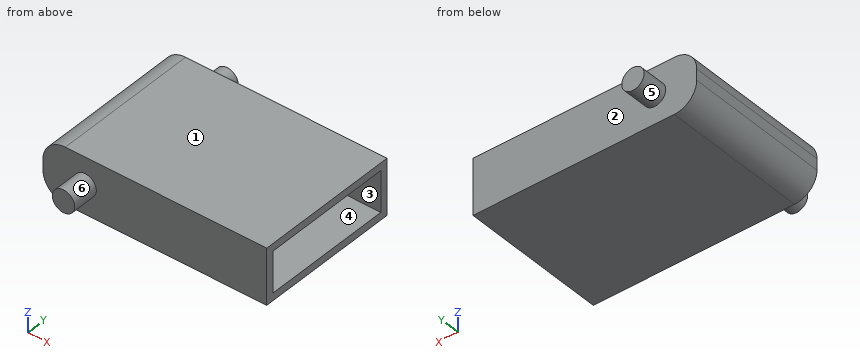
```python
from build123d import *

# Parameters (mm, degrees)
F1_DEPTH = 50
F2_T     = -2.54
F3_R     = 3.81
F4_DEPTH = 9
F5_R     = 3.81
F6_DEPTH = 9


with BuildPart() as f1:
    # F0 (on Front) → F1 (new body)
    with BuildSketch(Plane.XZ):
        with BuildLine():
            Line((31.366751, 9.340362), (-37.213249, 9.340362))
            ThreePointArc((-37.213249, 9.340362), (-42.601402, 7.108516), (-44.833249, 1.720362))
            Line((-44.833249, 1.720362), (-44.833249, -2.089638))
            ThreePointArc((-44.833249, -2.089638), (-42.601402, -7.477792), (-37.213249, -9.709638))
            Line((-37.213249, -9.709638), (31.366751, -9.709638))
            Line((31.366751, -9.709638), (31.366751, 9.340362))
        make_face()
    extrude(amount=F1_DEPTH)

    # F2
    f2_openings = [f1.faces().sort_by_distance(p)[0] for p in [
        (31.366751, -25, -0.184638),
    ]]
    offset(amount=F2_T, openings=f2_openings)

    # F3 (on face) → F4 (join)
    with BuildSketch(Plane.XZ.offset(50)):
        with Locations((-30.48, 0)):
            Circle(F3_R)
    extrude(amount=F4_DEPTH)

    # F5 (on face) → F6 (join)
    with BuildSketch(Plane(origin=(0, 0, 0), x_dir=(-1, 0, 0), z_dir=(0, 1, 0))):
        with Locations((30.48, 0)):
            Circle(F5_R)
    extrude(amount=F6_DEPTH)


solid = f1.part
```
Verification items for the finished model (mm, model axes). Face numbers are marked on the shaded views. A direction names the side the tool comes from. Coordinates: 2 decimals unless noted, no trailing zeros. Write each loop counter-clockwise with the first axis right and the second up, starting at its lowest first coordinate (ties: lowest second). Pieces come first, ordered by that corner, then holes. Notation, with made-up numbers: M 84,15 L 115,15 A19 cw 115,39 Z; hole C -9,-14.5 d10. An arc over 180 degrees is marked long. One line per item, written item: value.
Item 1: Access from +Z, -Z, +X, -X, +Y, -Y to the whole of each face (thin tool, end or side, straight path). Record for the marked faces 4, 5 and 6.
Check sheet entries:
face 4: +X
face 5: +Y
face 6: -Y
Item 2: Section check D-D, the plane x = -7. Record the boundary of the cut face in (y, z), plus the area to 3 significant figures.
Check sheet entries:
outline: M -50,-9.71 L 0,-9.71 L 0,9.34 L -50,9.34 Z; hole M -47.46,-7.17 L -2.54,-7.17 L -2.54,6.8 L -47.46,6.8 Z
area: 325 mm^2
Item 3: Section check C-C, the plane y = -19. Record the boundary of the cut face in (x, z).
Check sheet entries:
outline: M -44.83,-2.09 A7.62 ccw -37.21,-9.71 L 31.37,-9.71 L 31.37,-7.17 L -37.21,-7.17 A5.08 cw -42.29,-2.09 L -42.29,1.72 A5.08 cw -37.21,6.8 L 31.37,6.8 L 31.37,9.34 L -37.21,9.34 A7.62 ccw -44.83,1.72 Z
Item 4: Scan lines: line 1 along Y through (x, z) = (25, -0.5); line 2 along Z through (x, y) = (1, -10); line 3 along Y through (x, z) = (1, 7). Record each from-to range of solid material in increasing order.
Check sheet entries:
line 1: y = -50 to -47.46, -2.54 to 0
line 2: z = -9.71 to -7.17, 6.8 to 9.34
line 3: y = -50 to 0
Item 5: Section check B-B, the plane z = 0. Record the boundary of the cut face in (x, y), plus the area to 3 significant figures.
Check sheet entries:
outline: M -44.83,-50 L -34.29,-50 L -34.29,-59 L -26.67,-59 L -26.67,-50 L 31.37,-50 L 31.37,-47.46 L -42.29,-47.46 L -42.29,-2.54 L 31.37,-2.54 L 31.37,0 L -26.67,0 L -26.67,9 L -34.29,9 L -34.29,0 L -44.83,0 Z
area: 638 mm^2
Item 6: Section check A-A, the plane x = -30.48. Record the boundary of the cut face in (y, z), plus the area to 3 significant figures.
Check sheet entries:
outline: M -59,-3.81 L -50,-3.81 L -50,-9.71 L 0,-9.71 L 0,-3.81 L 9,-3.81 L 9,3.81 L 0,3.81 L 0,9.34 L -50,9.34 L -50,3.81 L -59,3.81 Z; hole M -47.46,-7.17 L -2.54,-7.17 L -2.54,6.8 L -47.46,6.8 Z
area: 462 mm^2
Item 7: Mould release check, pull along Y, two halves, no side actions. Record for the marked faces 1, 2 and 3: pulls with the +Y half, pulls with the -Y half, needs draft (parallel to the pull), parting line crosses it, or undercut.
Check sheet entries:
face 1: needs draft
face 2: pulls with the +Y half
face 3: undercut
Item 8: Gauge pin test, flat ends, axial feed: pin 1 Ø8 at (y, z) = (-41, -7.5) entering from -X; pin 2 Ø3 at (y, z) = (-29, -0.5) entering from +X; pin 3 Ø3 at (x, z) = (22.5, 2) entering from -Y. Record the tip position at first contact, or that the pin passes through.
Check sheet entries:
pin 1: stops at x = -44.7
pin 2: stops at x = -42.29
pin 3: stops at y = -50
